Geometry: see drawing. Coordinates: mm, zero at the bounding-box minimum. A direction names the side the tool comes from. Round coordinates to 2 decimals unless told otherwise and drop trailing zeros. Order: outer loops, then holes, each group sorted by start corner. A loop starts at its lowest first (then second) coordinate and runs counter-clockwise, first axis right, second up. Notation, with made-up numbers: (4.25, -40) -> (48.25, -40) arc R19 cw to (48.25, -19) -> close; hole circle Ø4 at (40.25, -12.5). An arc over 180 degrees is marked (long way). One line per item, written item: value. Start each with the question number.
1) Section C-C (x = 6.25). Return the cut outline in (y, z) (1 decimal).
2) Reachability of the marked faces 1 and 2 from +Z, -Z, +X, -X, +Y, -Y: full face, straight path, thin tool, end or side. Return the list, or none.
3) Section D-D (z = 28). Return the cut outline in (x, y).
4) Section B-B (z = 17). Return the cut outline in (x, y), and give its area (3 significant figures).
5) Section A-A (z = 10.5). Return the cut outline in (x, y) (1 decimal).
6) Ray query, L1, parallel to Z at x = 3.25, y = 5.75; L2, parallel to Y at x = 4, z = 28; L3, parallel to X at y = 1, z = 3.5 (1 decimal). Return the intervals inside material, ascending.
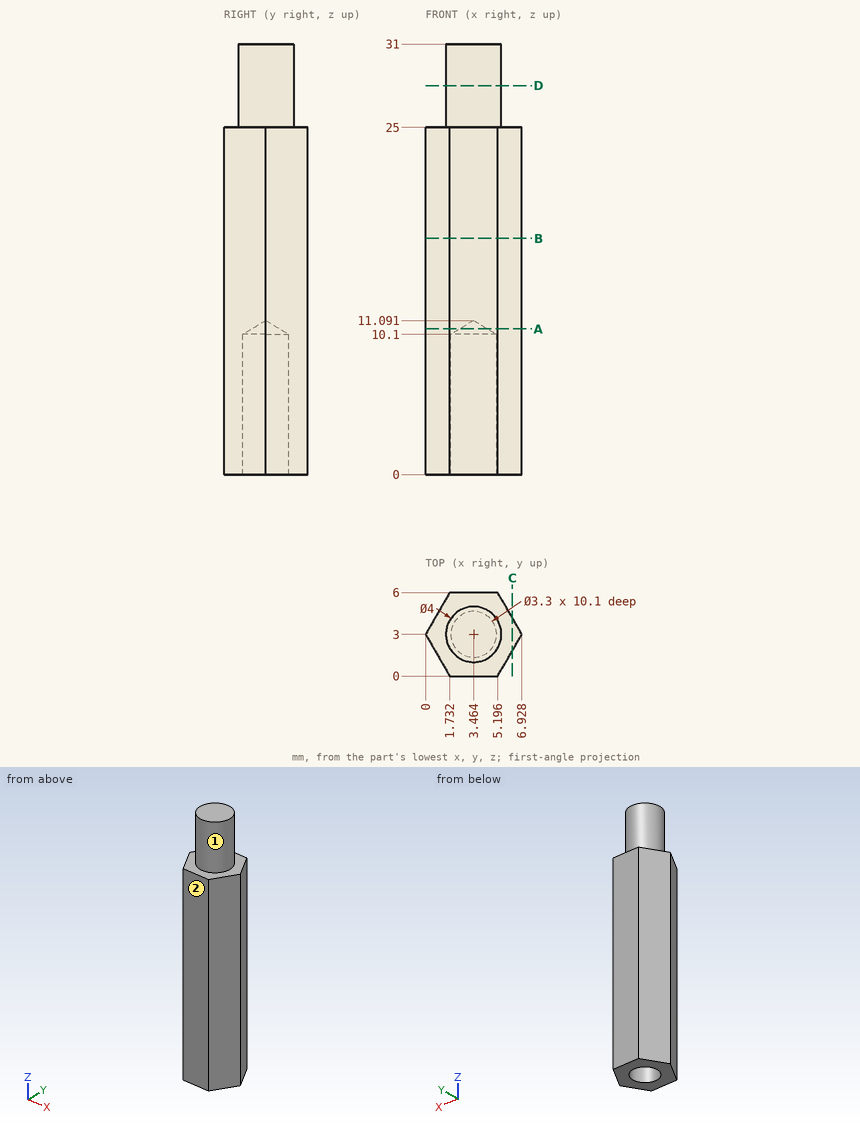
Findings:
1. outline: (1.8, 0) -> (4.2, 0) -> (4.2, 25) -> (1.8, 25) -> close
2. face 1: +Z
2. face 2: +Z, -Z, +X, -X, -Y
3. outline: circle Ø4 at (3.46, 3)
4. outline: (0, 3) -> (1.73, 0) -> (5.2, 0) -> (6.93, 3) -> (5.2, 6) -> (1.73, 6) -> close
4. area: 31.2 mm2
5. outline: (0, 3) -> (1.7, 0) -> (5.2, 0) -> (6.9, 3) -> (5.2, 6) -> (1.7, 6) -> close; hole circle Ø2 at (3.5, 3)
6. L1: 0 to 25
6. L2: 1.07 to 4.93
6. L3: 1.2 to 5.8
